Here's how the part is built. I have some questions about the finished solid (model axes, mm). Give positions to 0.01 mm unless a question says otherwise; leave off trailing zeros. Write each loop counter-clockwise with the first axis right and the second up, starting at its lowest first coordinate (ties: lowest second). Pieces come first, ordered by that corner, then holes. Notation, with made-up numbers: M -18,24.25 L 30,24.25 A14 ccw 30,32.25 Z; hole C 26,-17 d3. An arc over 180 degrees is marked long. Answer as CSV lines item,"result". Start each with the question number.
Q1. If I drill on line 1 along X through (y, z) = (-0.1, -0.3); line 2 along X through (y, z) = (0.7, -0.8); line 3 along Z through (x, y) = (10, -0.4), over which ranges is the centre line in solid material (lowest first)?
Q2. Suppose I cut it at A-A (z = 0). Write out the boundary of the cut face in (x, y), then the cut area to 3 significant figures.
Q3. Suppose I cut it at B-B (x = 19). Write out the boundary of the cut face in (y, z).
```python
from build123d import *

# Parameters (mm, degrees)
SKETCH2_W                    = 2.4892
SKETCH2_H                    = 0.4318
SLOT_DEPTH                   = 0.4572
SCHIZZO2_R                   = 0.5969
ESTRUSIONE_ESTRUSIONE1_DEPTH = 15.1257


with BuildPart() as part:
    # BodySke → Base-Revolve (revolve)
    with BuildSketch(Plane.XY):
        with BuildLine():
            Line((0.7112, 0.5969), (0.7112, 1.2446))
            Line((0.7112, 1.2446), (0.2794, 1.206822395))
            ThreePointArc((0.2794, 1.206822395), (0.070761718, 0.619371587), (0, 0))
            Line((0, 0), (16.5862, 0))
            Line((16.5862, 0), (16.5862, 0.5969))
            Line((16.5862, 0.5969), (0.7112, 0.5969))
        make_face()
    revolve(axis=Axis((-25.4, 0, 0), (1, 0, 0)))

    # Sketch2 → Slot (cut)
    with BuildSketch(Plane(origin=(0, 0, 0), x_dir=(0, 0, -1), z_dir=(1, 0, 0))):
        Rectangle(SKETCH2_W, SKETCH2_H)
    extrude(amount=SLOT_DEPTH, mode=Mode.SUBTRACT)

    # Schizzo2 → Estrusione-Estrusione1 (add)
    with BuildSketch(Plane(origin=(16.5862, 0, 0), x_dir=(0, 0, -1), z_dir=(1, 0, 0))):
        Circle(SCHIZZO2_R)
    extrude(amount=ESTRUSIONE_ESTRUSIONE1_DEPTH)


solid = part.part
```
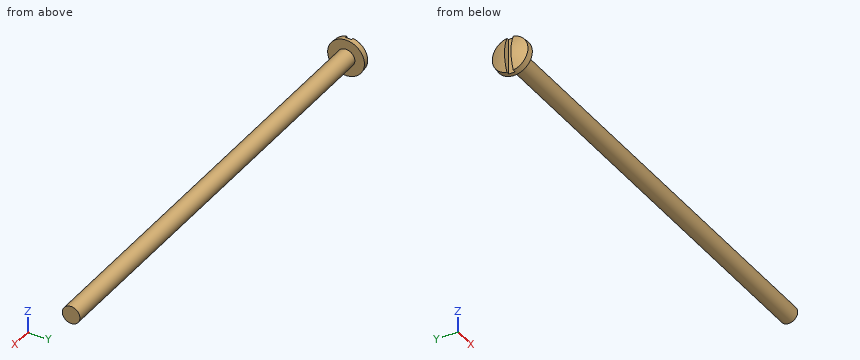
Resolved:
1,line 1,"0.46 to 31.71"
1,line 2,"0.21 to 0.71"
1,line 3,"-0.44 to 0.44"
2,outline,"M 0.01,-0.22 A2.75 ccw 0.28,-1.21 L 0.71,-1.24 L 0.71,-0.6 L 31.71,-0.6 L 31.71,0.6 L 0.71,0.6 L 0.71,1.24 L 0.28,1.21 A2.75 ccw 0.01,0.22 L 0.46,0.22 L 0.46,-0.22 Z"
2,area,"38.3 mm^2"
3,outline,"C 0,0 d1.19"
